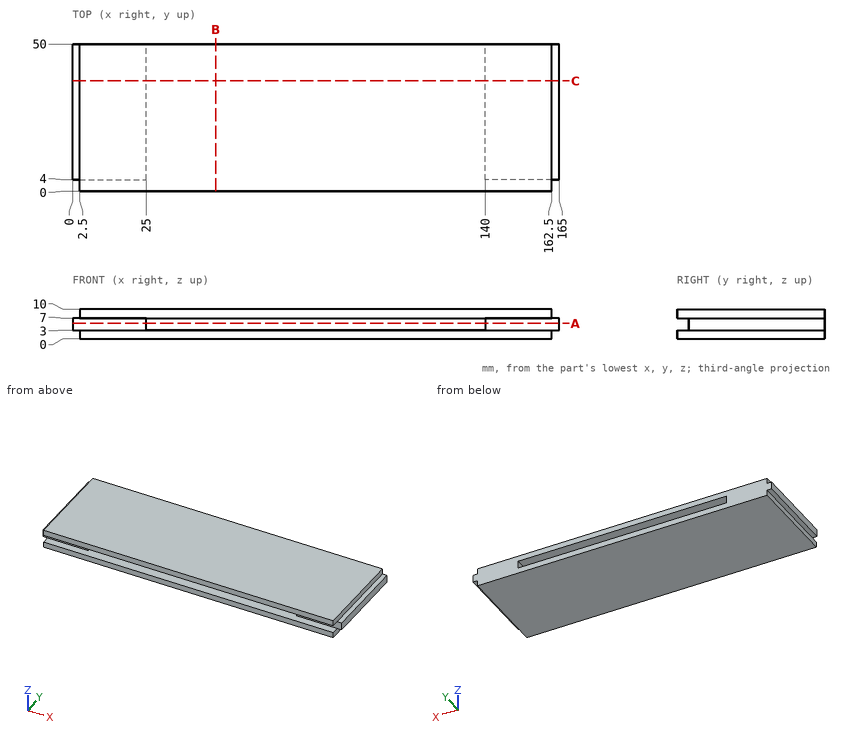
Source: three-view drawing plus pictorial views. Frame: mm from the lowest corner of the part. Coordinates: 2 decimals unless noted, no trailing zeros. Order: outer loops, then holes, each group sorted by start corner. A loop starts at its lowest first (then second) coordinate and runs counter-clockwise, first axis right, second up.
1) Ray query, probe 1 along Z at (x, y) = (119, 7); probe 2 along X at (y, z) = (38.5, 3.5); probe 3 along Y at (x, z) = (11.5, 3.25). Return the intervals inside material, ascending.
Result sheet:
probe 1: z = 0 to 3, 7 to 10
probe 2: x = 0 to 25, 140 to 165
probe 3: y = 4 to 50
2) Section B-B (x = 48.5). Return loops of the section in (y, z).
Result sheet:
outline: (0, 0) - (50, 0) - (50, 3) - (0, 3) - close; (0, 7) - (50, 7) - (50, 10) - (0, 10) - close
3) Section A-A (z = 5.25). Return loops of the section in (x, y).
Result sheet:
outline: (0, 4) - (25, 4) - (25, 50) - (0, 50) - close; (140, 4) - (165, 4) - (165, 50) - (140, 50) - close
4) Section C-C (y = 37.5). Return loops of the section in (x, z), then the cut area to 3 significant figures.
Result sheet:
outline: (0, 3) - (2.5, 3) - (2.5, 0) - (162.5, 0) - (162.5, 3) - (165, 3) - (165, 7) - (162.5, 7) - (162.5, 10) - (2.5, 10) - (2.5, 7) - (0, 7) - close; hole (25, 3) - (140, 3) - (140, 7) - (25, 7) - close
area: 1,160 mm2
5) First-contact query: P1, Ø3, axis at x = 22.5, y = 37, coming from the -Z side; P2, Ø1.5, axis at y = 17, z = 9, coming from the +X side; P3, Ø1.2, axis at x = 157, z = 5, coming from the -Y side; P4, Ø2, axis at x = 164, y = 29, coming from the -Z side. Flat tips, straight axial feed; report the tip coordinate or a pass-through.
Result sheet:
P1: stops at z = 0
P2: stops at x = 162.5
P3: stops at y = 4
P4: stops at z = 3
